Can you work these out from the drawing? Everything is in mm from the part's minimum corner. A direction names the side the tool comes from. Coordinates: 2 decimals unless noted, no trailing zeros. Write each loop counter-clockwise with the first axis right and the second up, starting at its lowest first coordinate (ties: lowest second). Pieces come first, ordered by that corner, then holes.
(1) Imagine slicing it at C-C, the plane x = 25. List the corners of the cut face in (y, z) for me, plus the area to 3 significant figures.
(2) Which directions (+Z, -Z, +X, -X, +Y, -Y) give clear straight access to the entire face, cutting with the end or side of a thin tool? Please do the marked faces 1 and 2.
(3) Imagine slicing it at A-A, the plane y = 15. List the corners of the cut face in (x, z) for me.
(4) Imagine slicing it at D-D, the plane y = 23. List the corners of the cut face in (x, z) for me (1 decimal).
(5) Please list where these lines run through material, in increasing order: probe 1 along Y at (x, z) = (15, 13.9); probe 2 along Z at (x, y) = (11.75, 9.75).
(6) Thinking about a two-plate mould opening in X: for the marked faces 3, 4 and 5, which applies, released by +X, released by -X, zero draft, split by the parting line, or undercut?
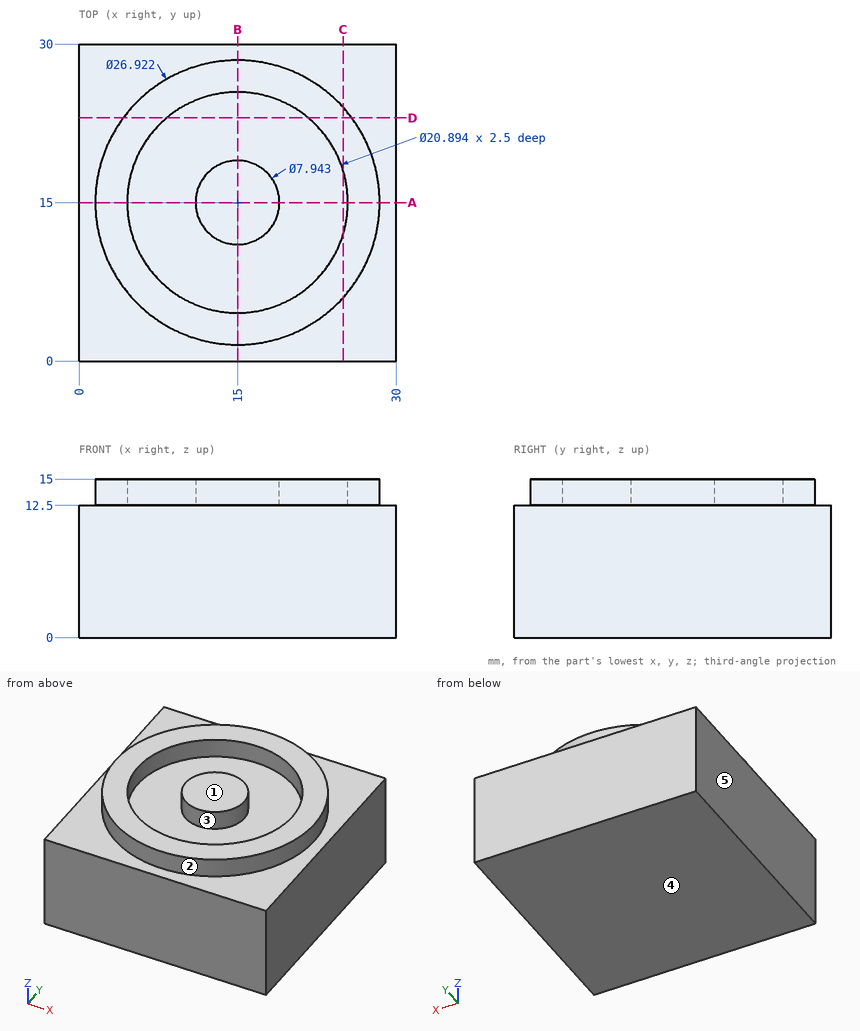
Recorded:
1. outline: (0, 0) - (30, 0) - (30, 12.5) - (24.01, 12.5) - (24.01, 15) - (18.02, 15) - (18.02, 12.5) - (11.98, 12.5) - (11.98, 15) - (5.99, 15) - (5.99, 12.5) - (0, 12.5) - close
1. area: 405 mm2
2. face 1: +Z, +X, -X, +Y, -Y
2. face 2: +Z
3. outline: (0, 0) - (30, 0) - (30, 12.5) - (28.46, 12.5) - (28.46, 15) - (25.45, 15) - (25.45, 12.5) - (18.97, 12.5) - (18.97, 15) - (11.03, 15) - (11.03, 12.5) - (4.55, 12.5) - (4.55, 15) - (1.54, 15) - (1.54, 12.5) - (0, 12.5) - close
4. outline: (0, 0) - (30, 0) - (30, 12.5) - (25.8, 12.5) - (25.8, 15) - (21.7, 15) - (21.7, 12.5) - (8.3, 12.5) - (8.3, 15) - (4.2, 15) - (4.2, 12.5) - (0, 12.5) - close
5. probe 1: y = 1.54 to 4.55, 11.03 to 18.97, 25.45 to 28.46
5. probe 2: z = 0 to 12.5
6. face 3: undercut
6. face 4: zero draft
6. face 5: released by -X
